Geometry check sheet. Reference: the model listing, model coordinates, mm. A direction names the side the tool comes from. Give positions to 0.01 mm unless a question says otherwise; leave off trailing zeros. Order: outer loops, then holes, each group sorted by start corner. A loop starts at its lowest first (then second) coordinate and runs counter-clockwise, first axis right, second up. Notation, with made-up numbers: (-7, 39) - (34, 39) arc R17 cw to (34, 68) - close; hole circle Ø3 at (-31.75, 47). An arc over 180 degrees is marked (long way). Put each result on its own line as item: value. Start each with the question number.
```python
from build123d import *

# Parameters (mm, degrees)
STOCK_FULL_SHAPE_1_OUTLINE_W     = 110
STOCK_FULL_SHAPE_1_OUTLINE_H     = 50
STOCK_FULL_SHAPE_1_DEPTH         = 2
STOCK_FULL_START                 = 2
STOCK_FULL_SHAPE_1_2_OUTLINE_W   = 110
STOCK_FULL_SHAPE_1_2_OUTLINE_H   = 50
STOCK_FULL_SHAPE_1_2_OUTLINE_W_2 = 107
STOCK_FULL_SHAPE_1_2_OUTLINE_H_2 = 47
STOCK_FULL_SHAPE_1_2_DEPTH       = 3
BOSS_EXTRUDE1_DEPTH              = 10
BOSS_EXTRUDE2_DEPTH              = 10
BOSS_EXTRUDE3_DEPTH              = 10
BOSS_EXTRUDE4_DEPTH              = 10
CUT_EXTRUDE3_DEPTH               = 7
SKETCH9_W                        = 106.6
SKETCH9_H                        = 2
CUT_EXTRUDE4_DEPTH               = 87
SKETCH10_W                       = 7.6
SKETCH10_H                       = 1.5
CUT_EXTRUDE5_DEPTH               = 3
SKETCH11_W                       = 110
SKETCH11_H                       = 50
BOSS_EXTRUDE5_DEPTH              = 2
BOSS_EXTRUDE6_DEPTH              = 2
SKETCH13_W                       = 7.6
SKETCH13_H                       = 1.5
CUT_EXTRUDE6_DEPTH               = 0.1
SKETCH1_W                        = 13.5
SKETCH1_H                        = 1.5
CUT_EXTRUDE7_DEPTH               = 10.1
FILLET1_R                        = 2


# Read off the part's stored shape, not the designer's step: Stock-full shape-1
with BuildPart() as part:
    # Stock-full shape-1 outline → Stock-full shape-1 (new body)
    with BuildSketch(Plane(origin=(0, 0, 0), x_dir=(1, 0, 0), z_dir=(0, 1, 0))):
        with Locations((14.090909091, -5.886363636)):
            Rectangle(STOCK_FULL_SHAPE_1_OUTLINE_W, STOCK_FULL_SHAPE_1_OUTLINE_H)
    extrude(amount=STOCK_FULL_SHAPE_1_DEPTH)

    # Stock-full shape-1 2 outline → Stock-full shape-1 2 (add)
    with BuildSketch(Plane(origin=(0, 0, 0), x_dir=(1, 0, 0), z_dir=(0, 1, 0)).offset(STOCK_FULL_START)):
        with Locations((14.090909091, -5.886363636)):
            Rectangle(STOCK_FULL_SHAPE_1_2_OUTLINE_W, STOCK_FULL_SHAPE_1_2_OUTLINE_H)
        with Locations((14.090909091, -5.886363636)):
            Rectangle(STOCK_FULL_SHAPE_1_2_OUTLINE_W_2, STOCK_FULL_SHAPE_1_2_OUTLINE_H_2, mode=Mode.SUBTRACT)
    extrude(amount=STOCK_FULL_SHAPE_1_2_DEPTH)

    # Sketch4 → Boss-Extrude1 (add)
    with BuildSketch(Plane(origin=(0, 2, 0), x_dir=(1, 0, 0), z_dir=(0, 1, 0))):
        Polygon((-39.409090909, 12.824440082), (-39.409090909, 17.613636364), (-34.409090909, 17.613636364), (-34.409090909, 15.913636364), (-37.709090909, 15.913636364), (-37.709090909, 12.613636364), (-39.409090909, 12.613636364), align=None)
    extrude(amount=BOSS_EXTRUDE1_DEPTH)

    # Sketch5 → Boss-Extrude2 (add)
    with BuildSketch(Plane(origin=(0, 2, 0), x_dir=(1, 0, 0), z_dir=(0, 1, 0))):
        Polygon((-39.409090909, -29.386363636), (-39.409090909, -24.386363636), (-37.709090909, -24.386363636), (-37.709090909, -27.686363636), (-34.409090909, -27.686363636), (-34.409090909, -29.386363636), align=None)
    extrude(amount=BOSS_EXTRUDE2_DEPTH)

    # Sketch6 → Boss-Extrude3 (add)
    with BuildSketch(Plane(origin=(0, 2, 0), x_dir=(1, 0, 0), z_dir=(0, 1, 0))):
        Polygon((67.590909091, 17.613636364), (62.590909091, 17.613636364), (62.590909091, 15.913636364), (65.890909091, 15.913636364), (65.890909091, 12.613636364), (67.590909091, 12.613636364), align=None)
    extrude(amount=BOSS_EXTRUDE3_DEPTH)

    # Sketch7 → Boss-Extrude4 (add)
    with BuildSketch(Plane(origin=(0, 2, 0), x_dir=(1, 0, 0), z_dir=(0, 1, 0))):
        Polygon((67.590909091, -24.386363636), (67.590909091, -29.386363636), (62.590909091, -29.386363636), (62.590909091, -27.686363636), (65.890909091, -27.686363636), (65.890909091, -24.386363636), align=None)
    extrude(amount=BOSS_EXTRUDE4_DEPTH)

    # Sketch8 → Cut-Extrude3 (cut)
    with BuildSketch(Plane(origin=(0, 12, 0), x_dir=(1, 0, 0), z_dir=(0, 1, 0))):
        Polygon((62.590909091, -29.386363636), (62.590909091, -29.186363636), (67.390909091, -29.186363636), (67.390909091, -24.386363636), (67.590909091, -24.386363636), (67.590909091, -29.386363636), align=None)
        Polygon((62.590909091, 17.613636364), (62.590909091, 17.413636364), (67.390909091, 17.413636364), (67.390909091, 12.613636364), (67.590909091, 12.613636364), (67.590909091, 17.613636364), align=None)
        Polygon((-39.409090909, 12.613636364), (-39.409090909, 17.613636364), (-34.409090909, 17.613636364), (-34.409090909, 17.413636364), (-39.209090909, 17.413636364), (-39.209090909, 12.613636364), align=None)
        Polygon((-39.409090909, -24.386363636), (-39.409090909, -29.386363636), (-34.409090909, -29.386363636), (-34.409090909, -29.186363636), (-39.209090909, -29.186363636), (-39.209090909, -24.386363636), align=None)
    extrude(amount=-CUT_EXTRUDE3_DEPTH, mode=Mode.SUBTRACT)

    # Sketch9 → Cut-Extrude4 (cut)
    with BuildSketch(Plane.XY.offset(29.186363636)):
        with Locations((14.090909091, 11)):
            Rectangle(SKETCH9_W, SKETCH9_H)
    extrude(amount=-CUT_EXTRUDE4_DEPTH, mode=Mode.SUBTRACT)

    # Sketch10 → Cut-Extrude5 (cut)
    with BuildSketch(Plane(origin=(0, 5, 0), x_dir=(1, 0, 0), z_dir=(0, 1, 0))):
        with Locations((-27.409090909, -30.136363636)):
            Rectangle(SKETCH10_W, SKETCH10_H)
    extrude(amount=-CUT_EXTRUDE5_DEPTH, mode=Mode.SUBTRACT)

    # Sketch11 → Boss-Extrude5 (add)
    with BuildSketch(Plane(origin=(0, 5, 0), x_dir=(1, 0, 0), z_dir=(0, 1, 0))):
        with Locations((14.090909091, -5.886363636)):
            Rectangle(SKETCH11_W, SKETCH11_H)
        Polygon((-39.209090909, 17.413636364), (-39.209090909, 12.613636364), (-39.409090909, 12.613636364), (-39.409090909, -24.386363636), (-39.209090909, -24.386363636), (-39.209090909, -29.186363636), (-34.409090909, -29.186363636), (-34.409090909, -29.386363636), (-31.209090909, -29.386363636), (62.590909091, -29.386363636), (62.590909091, -29.186363636), (67.390909091, -29.186363636), (67.390909091, -24.386363636), (67.590909091, -24.386363636), (67.590909091, 12.613636364), (67.390909091, 12.613636364), (67.390909091, 17.413636364), (62.590909091, 17.413636364), (62.590909091, 17.613636364), (-34.409090909, 17.613636364), (-34.409090909, 17.413636364), align=None, mode=Mode.SUBTRACT)
    extrude(amount=BOSS_EXTRUDE5_DEPTH)

    # Sketch12 → Boss-Extrude6 (add)
    with BuildSketch(Plane(origin=(0, 10, 0), x_dir=(1, 0, 0), z_dir=(0, 1, 0))):
        Polygon((-37.709090909, -24.386363636), (-39.209090909, -24.386363636), (-39.209090909, -29.186363636), (-34.409090909, -29.186363636), (-34.409090909, -27.686363636), (-37.709090909, -27.686363636), align=None)
        Polygon((62.590909091, -29.186363636), (67.390909091, -29.186363636), (67.390909091, -24.386363636), (65.890909091, -24.386363636), (65.890909091, -27.686363636), (62.590909091, -27.686363636), align=None)
        Polygon((67.390909091, 12.613636364), (65.890909091, 12.613636364), (65.890909091, 15.913636364), (62.590909091, 15.913636364), (62.590909091, 17.413636364), (67.390909091, 17.413636364), align=None)
        Polygon((-37.709090909, 12.613636364), (-39.209090909, 12.613636364), (-39.209090909, 17.413636364), (-34.409090909, 17.413636364), (-34.409090909, 15.913636364), (-37.709090909, 15.913636364), align=None)
    extrude(amount=BOSS_EXTRUDE6_DEPTH)

    # Sketch13 → Cut-Extrude6 (cut)
    with BuildSketch(Plane.XZ.offset(-5)):
        with Locations((-27.409090909, 30.136363636)):
            Rectangle(SKETCH13_W, SKETCH13_H)
    extrude(amount=-CUT_EXTRUDE6_DEPTH, mode=Mode.SUBTRACT)

    # Sketch1 → Cut-Extrude7 (cut)
    with BuildSketch(Plane(origin=(0, 5, 0), x_dir=(1, 0, 0), z_dir=(0, 1, 0))):
        with Locations((48.140909091, -30.136363636)):
            Rectangle(SKETCH1_W, SKETCH1_H)
    extrude(amount=CUT_EXTRUDE7_DEPTH, mode=Mode.SUBTRACT)

    # Fillet1
    fillet1_edges = [part.edges().sort_by_distance(p)[0] for p in [
        (-40.909090909, 2.5, -19.113636364),
        (69.090909091, 2.5, -19.113636364),
        (69.090909091, 2.5, 30.886363636),
        (-40.909090909, 2.5, 30.886363636),
    ]]
    fillet(fillet1_edges, radius=FILLET1_R)


solid = part.part
```
Item 1: Cross-section at A-A (y = 9.75). Enter the section's corners in (x, z).
Item 2: Thickness scan on line 1 along X through (y, z) = (5.25, -12.5); line 2 along Z through (x, y) = (9, 5); line 3 along Y through (x, z) = (62.5, 18). Record the ranges inside material, lowest first.
Item 3: Set-up check for faces 1 (the face through (15, 4, 29.386)), 2 (the face through (-39.209, 10, -15)), 3 (the face through (-37, 9, 29.186)), 4 (the face through (-37, 10, -17.414)), 5 (the face through (65, 12, 28)): record each of +Z, -Z, +X, -X, +Y, -Y from which the full face is reachable in a straight line by a thin tool's end or side.
Item 4: Cross-section at D-D (x = 38). Enter the section's corners in (y, z), and give its area (3 significant figures).
Item 5: Cross-section at B-B (x = -27). Enter the section's corners in (y, z).
Item 6: Release check for a two-part mould opening along X. For faces 6 (the face through (68.521, 3.549, 30.285)), 7 (the face through (64, 7, -15.914)), 8 (the face through (65, 10, 29.186)) record: +X half, -X half, draft (parallel to the pull), parting line (faces both ways), or undercut.
Item 7: Gauge pin test, flat ends, axial feed: pin 1 Ø2.5 at (x, y) = (64.5, 10) entering from -Z; pin 2 Ø1.6 at (y, z) = (5.5, 30) entering from +X; pin 3 Ø0.8 at (y, z) = (3.5, 30.5) entering from -X; pin 4 Ø4 at (x, y) = (38, 10) entering from -Z. Record the tip position at first contact, or that the pin passes through.
Recorded:
1. outline: (-39.21, -17.41) - (-34.41, -17.41) - (-34.41, -15.91) - (-37.71, -15.91) - (-37.71, -12.61) - (-39.21, -12.61) - close; (-39.21, 24.39) - (-37.71, 24.39) - (-37.71, 27.69) - (-34.41, 27.69) - (-34.41, 29.19) - (-39.21, 29.19) - close; (62.59, -17.41) - (67.39, -17.41) - (67.39, -12.61) - (65.89, -12.61) - (65.89, -15.91) - (62.59, -15.91) - close; (62.59, 27.69) - (65.89, 27.69) - (65.89, 24.39) - (67.39, 24.39) - (67.39, 29.19) - (62.59, 29.19) - close
2. line 1: x = -40.91 to -39.41, 67.59 to 69.09
2. line 2: z = -19.11 to -17.61, 29.39 to 30.89
2. line 3: y = 0 to 2
3. face 1: +Y
3. face 2: +Z, -Z, -X, +Y
3. face 3: +Z, +X, -X, +Y
3. face 4: -Z, +X, -X, +Y
3. face 5: +Z, -Z, +X, -X, +Y
4. outline: (0, -19.11) - (7, -19.11) - (7, -17.61) - (2, -17.61) - (2, 29.39) - (7, 29.39) - (7, 30.89) - (0, 30.89) - close
4. area: 115 mm^2
5. outline: (0, -19.11) - (7, -19.11) - (7, -17.61) - (2, -17.61) - (2, 30.89) - (0, 30.89) - close; (5.1, 29.39) - (7, 29.39) - (7, 30.89) - (5.1, 30.89) - close
6. face 6: +X half
6. face 7: undercut
6. face 8: draft
7. pin 1: stops at z = -17.41
7. pin 2: stops at x = 69.07
7. pin 3: stops at x = -40.5
7. pin 4: passes through
